```python
from build123d import *

# Parameters (mm, degrees)
SKETCH1_R           = 78.232
SKETCH1_R_2         = 76.2
BOSS_EXTRUDE1_DEPTH = 406.4
CUT_EXTRUDE1_DEPTH  = 0.381
CIRPATTERN1_COUNT   = 4


with BuildPart() as part:
    # Sketch1 → Boss-Extrude1 (new body)
    with BuildSketch(Plane(origin=(0, 0, 0), x_dir=(1, 0, 0), z_dir=(0, 1, 0))):
        with Locations(Location((0, 0, 0), (0, 0, 270))):
            Circle(SKETCH1_R)
        with Locations(Location((0, 0, 0), (0, 0, 270))):
            Circle(SKETCH1_R_2, mode=Mode.SUBTRACT)
    extrude(amount=BOSS_EXTRUDE1_DEPTH)

    # Sketch2 → Cut-Extrude1 (cut)
    with BuildSketch(Plane(origin=(78.232, 0, 0), x_dir=(0, 0, -1), z_dir=(1, 0, 0))):
        Polygon((0, 406.4), (6.35, 406.4), (6.35, 50.8), (-6.35, 50.8), (-6.35, 406.4), align=None)
    cut_extrude1 = extrude(amount=-CUT_EXTRUDE1_DEPTH, mode=Mode.SUBTRACT)

    # CirPattern1: Cut-Extrude1 ×4 about axis
    cirpattern1_axis = Axis((0, 0, 0), (0, 1, 0))
    for i in range(1, CIRPATTERN1_COUNT):
        add(cut_extrude1.rotate(cirpattern1_axis, i * 360 / CIRPATTERN1_COUNT), mode=Mode.SUBTRACT)


solid = part.part
```
The listing builds one solid part. Answer for the finished solid, in the listing's coordinates (mm). Round coordinates to 2 decimals unless told otherwise and drop trailing zeros. Order: outer loops, then holes, each group sorted by start corner. A loop starts at its lowest first (then second) coordinate and runs counter-clockwise, first axis right, second up. Notation, with made-up numbers: (12, 80.5) - (30, 80.5) arc R23 cw to (30, 117.5) - close; hole circle Ø11 at (-2, 67). An arc over 180 degrees is marked (long way). Put each result on its own line as item: value. Start each with the question number.
(1) Find section A-A (z = 0). Give the vertices of the cut face in (x, y), plus the area to 3 significant figures.
(2) Find section D-D (z = 29.5). Give the vertices of the cut face in (x, y).
(3) Find section B-B (y = 58.5). Give the vertices of the cut face in (x, z), plus the area to 3 significant figures.
(4) Straight lines are drawn through the part: probe 1 along X at (y, z) = (100, -3); probe 2 along X at (y, z) = (224, 0); probe 3 along Z at (x, y) = (14, 63). For each, find the intervals that lie inside material, in ascending order. Write a range as from..to.
(5) Find section C-C (x = 0). Give the vertices of the cut face in (y, z), plus the area to 3 significant figures.
(6) Given P1, Ø2, axis at x = -24.5, y = 88.5, coming from the +Z side; P2, Ø6, axis at x = -27.5, y = 195, coming from the +Z side; P3, Ø10, axis at y = 259, z = 1.5, coming from the -X side, each flat-ended and moving along its own axis, determine where each tip first touches the part or whether it passes through.
(7) Determine the mould class of faces 1 (the flat face through (-17, 406.4, 75)), 2 (the flat face through (0, 231, 77.851)), 3 (the cylindrical face through (23.5, 200.36, 74.62)), 4 (the cylindrical face through (-46.367, 200.355, -60.47)) for opening direction Z: released by +Z, released by -Z, zero draft, split by the parting line, or undercut.
Reply:
1. outline: (-78.23, 0) - (-76.2, 0) - (-76.2, 406.4) - (-77.85, 406.4) - (-77.85, 50.8) - (-78.23, 50.8) - close; (76.2, 0) - (78.23, 0) - (78.23, 50.8) - (77.85, 50.8) - (77.85, 406.4) - (76.2, 406.4) - close
1. area: 1,380 mm^2
2. outline: (-72.46, 0) - (-70.26, 0) - (-70.26, 406.4) - (-72.46, 406.4) - close; (70.26, 0) - (72.46, 0) - (72.46, 406.4) - (70.26, 406.4) - close
3. outline: (-77.97, -6.35) arc R78.23 ccw to (-6.35, -77.97) - (-6.35, -77.85) - (6.35, -77.85) - (6.35, -77.97) arc R78.23 ccw to (77.97, -6.35) - (77.85, -6.35) - (77.85, 6.35) - (77.97, 6.35) arc R78.23 ccw to (6.35, 77.97) - (6.35, 77.85) - (-6.35, 77.85) - (-6.35, 77.97) arc R78.23 ccw to (-77.97, 6.35) - (-77.85, 6.35) - (-77.85, -6.35) - close; hole circle Ø152.4 at (0, 0)
3. area: 971 mm^2
4. probe 1: -77.85..-76.14, 76.14..77.85
4. probe 2: -77.85..-76.2, 76.2..77.85
4. probe 3: -76.97..-74.9, 74.9..76.97
5. outline: (0, -78.23) - (50.8, -78.23) - (50.8, -77.85) - (406.4, -77.85) - (406.4, -76.2) - (0, -76.2) - close; (0, 76.2) - (406.4, 76.2) - (406.4, 77.85) - (50.8, 77.85) - (50.8, 78.23) - (0, 78.23) - close
5. area: 1,380 mm^2
6. P1: z = 74.62
6. P2: z = 74.3
6. P3: x = -77.97
7. face 1: zero draft
7. face 2: released by +Z
7. face 3: split by the parting line
7. face 4: undercut
